Check sheet for the drawn part. Datum: minimum x, y, z corner. Units: mm. Round coordinates to 2 decimals unless told otherwise and drop trailing zeros. Loops run counter-clockwise (first coordinate to the right, second up) from the corner with the lowest first, then second, coordinate; pieces in that order, holes last.
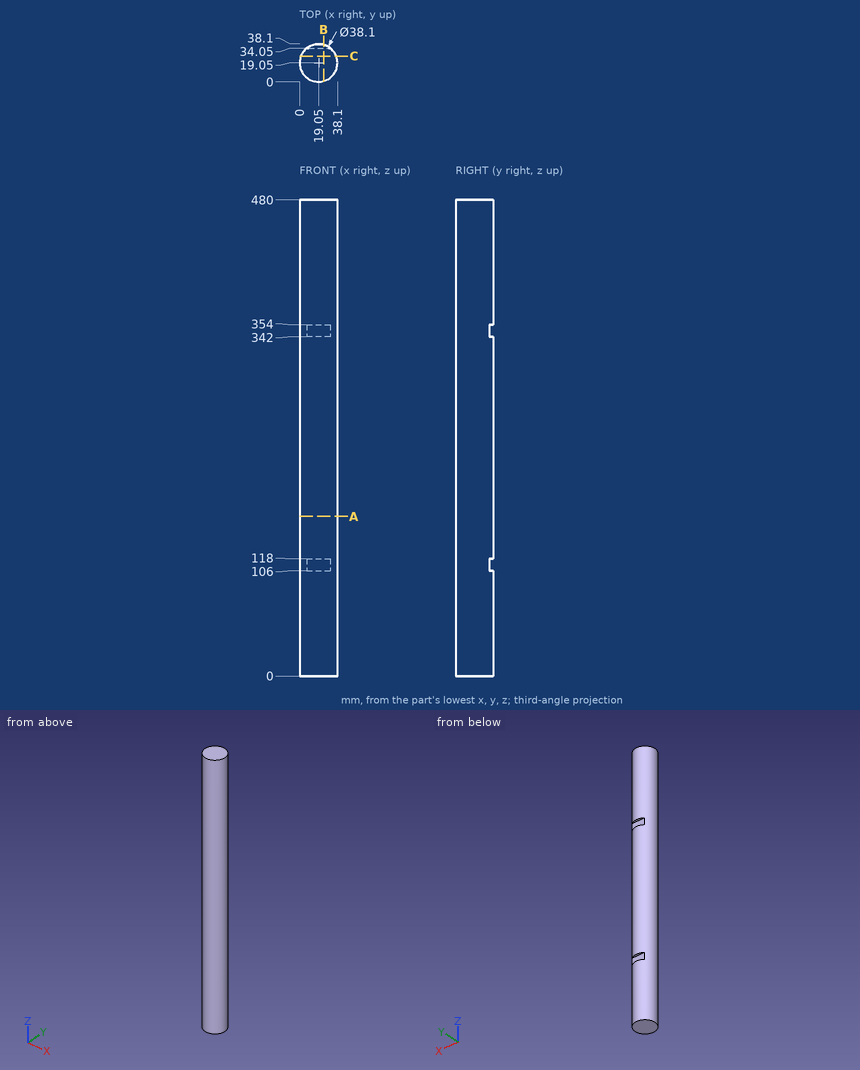
1) Sectioned sample at C-C, the plane y = 26. Record the cut outline in (x, z), then the cut area to 3 significant figures.
Report:
outline: (1.31, 0) - (36.79, 0) - (36.79, 480) - (1.31, 480) - close
area: 17,000 mm2
2) Gauge pin test, flat ends, axial feed: pin 1 (13 mm diameter, centred on x = 24.5, z = 349.5, fed in from +Y); pin 2 (1 mm diameter, centred on y = 9, z = 430.5, fed in from -X); pin 3 (6 mm diameter, centred on x = 19, z = 293.5, fed in from -Y). Record the tip position at first contact, or that the pin passes through.
Report:
pin 1: stops at y = 38.08
pin 2: stops at x = 2.57
pin 3: stops at y = 0
3) Scan lines: line 1 along X through (y, z) = (20.5, 206.5); line 2 along Y through (x, z) = (22.5, 217) (3 decimals); line 3 along Y through (x, z) = (6.5, 52.5). Record each from-to range of solid material in increasing order.
Report:
line 1: x = 0.06 to 38.04
line 2: y = 0.315 to 37.785
line 3: y = 4.72 to 33.38
4) Sectioned sample at A-A, the plane z = 161. Record the cut outline in (x, y), then the cut area to 3 significant figures.
Report:
outline: circle Ø38.1 at (19.05, 19.05)
area: 1,140 mm2
5) Sectioned sample at B-B, the plane x = 24. Record the cut outline in (y, z), then the cut area to 3 significant figures.
Report:
outline: (0.65, 0) - (37.45, 0) - (37.45, 106) - (34.05, 106) - (34.05, 118) - (37.45, 118) - (37.45, 342) - (34.05, 342) - (34.05, 354) - (37.45, 354) - (37.45, 480) - (0.65, 480) - close
area: 17,600 mm2
